Could you check a few things on this model? Use its own coordinates, in mm. A direction names the side the tool comes from. Round coordinates to 2 decimals unless told otherwise and drop trailing zeros. Loops run counter-clockwise (first coordinate to the right, second up) from the corner with the lowest first, then second, coordinate; pieces in that order, holes last. Notation, with made-up numbers: (70.5, 80.5) -> (115.5, 80.5) arc R31 ccw to (115.5, 112.5) -> close; hole circle Ø8 at (82, 53.5). An arc over 180 degrees is marked (long way). One line per item, written item: value.
from build123d import *

# Parameters (mm, degrees)
F0_W     = 406.4
F0_H     = 533.4
F1_DEPTH = 25.4
F2_W     = 306.07
F2_H     = 379.095
F3_DEPTH = 12.7
F4_R     = 12.7
F6_DEPTH = 6.35


with BuildPart() as f1:
    # F0 (on Top) → F1 (new body)
    with BuildSketch(Plane.XY):
        Rectangle(F0_W, F0_H)
    extrude(amount=F1_DEPTH)

    # F2 (on face) → F3 (cut)
    with BuildSketch(Plane.XY.offset(25.4)):
        Rectangle(F2_W, F2_H)
    extrude(amount=-F3_DEPTH, mode=Mode.SUBTRACT)

    # F4
    f4_edges = [f1.edges().sort_by_distance(p)[0] for p in [
        (-203.2, -266.7, 12.7),
        (203.2, -266.7, 12.7),
        (203.2, 266.7, 12.7),
        (-203.2, 266.7, 12.7),
        (-153.035, 189.5475, 19.05),
        (153.035, 189.5475, 19.05),
        (153.035, -189.5475, 19.05),
        (-153.035, -189.5475, 19.05),
    ]]
    fillet(f4_edges, radius=F4_R)

    # F5 (on face) → F6 (cut)
    with BuildSketch(Plane.XY.offset(25.4)):
        with BuildLine():
            Line((-196.85, 254), (-196.85, -254))
            ThreePointArc((-196.85, -254), (-194.990128, -258.490128), (-190.5, -260.35))
            Line((-190.5, -260.35), (190.5, -260.35))
            ThreePointArc((190.5, -260.35), (194.990128, -258.490128), (196.85, -254))
            Line((196.85, -254), (196.85, 254))
            ThreePointArc((196.85, 254), (194.990128, 258.490128), (190.5, 260.35))
            Line((190.5, 260.35), (-190.5, 260.35))
            ThreePointArc((-190.5, 260.35), (-194.990128, 258.490128), (-196.85, 254))
        make_face()
        with BuildLine():
            ThreePointArc((-187.325, -257.175), (-191.815128, -255.315128), (-193.675, -250.825))
            Line((-193.675, -250.825), (-193.675, 250.825))
            ThreePointArc((-193.675, 250.825), (-191.815128, 255.315128), (-187.325, 257.175))
            Line((-187.325, 257.175), (187.325, 257.175))
            ThreePointArc((187.325, 257.175), (191.815128, 255.315128), (193.675, 250.825))
            Line((193.675, 250.825), (193.675, -250.825))
            ThreePointArc((193.675, -250.825), (191.815128, -255.315128), (187.325, -257.175))
            Line((187.325, -257.175), (-187.325, -257.175))
        make_face(mode=Mode.SUBTRACT)
    extrude(amount=-F6_DEPTH, mode=Mode.SUBTRACT)


solid = f1.part
(1) If I drill on L1, parallel to X at y = 49, z = 19.5 (3 decimals); L2, parallel to Y at x = 107.5, z = 17.75; L3, parallel to X at y = 47.5, z = 18 (3 decimals), over which ranges is the centre line in solid material (lowest first)?
Recorded:
L1: -203.2 to -196.85, -193.675 to -153.035, 153.035 to 193.675, 196.85 to 203.2
L2: -266.7 to -189.55, 189.55 to 266.7
L3: -203.2 to -153.035, 153.035 to 203.2
(2) I'm going to push a flat-ended pin straight in: pin 1 Ø8 at (x, y) = (82, -21.5) entering from +Z. Where does the tip first touch, or does it pass through?
Recorded:
pin 1: z = 12.7
(3) If we section it at B-B, the plane y = 141: Please give me the cut outline in (x, z) (3 decimals), then the cut area to 3 significant figures.
Recorded:
outline: (-203.2, 0) -> (203.2, 0) -> (203.2, 25.4) -> (196.85, 25.4) -> (196.85, 19.05) -> (193.675, 19.05) -> (193.675, 25.4) -> (153.035, 25.4) -> (153.035, 12.7) -> (-153.035, 12.7) -> (-153.035, 25.4) -> (-193.675, 25.4) -> (-193.675, 19.05) -> (-196.85, 19.05) -> (-196.85, 25.4) -> (-203.2, 25.4) -> close
area: 6,400 mm²
(4) For faces 5 (the face through (169, 4, 25.4)), 6 (the face through (-2, -189.548, 19)), which set-ups out of +Z, -Z, +X, -X, +Y, -Y let a thin tool reach every point of the face, with its end or its side?
Recorded:
face 5: +Z, +X, -X, +Y, -Y
face 6: +Z
(5) Thinking about a two-plate mould opening in X: for faces 1 (the face through (-153.035, -2, 19)), 2 (the face through (-199.58, 262.88, 12.88)), 3 (the face through (203.2, -4, 13)), 4 (the face through (153.035, -2, 19)), which applies, released by +X, released by -X, zero draft, split by the parting line, or undercut?
Recorded:
face 1: undercut
face 2: released by -X
face 3: released by +X
face 4: undercut
